Read the model definition and answer for the solid it produces. Units are mm, in the model's axes. Face numbers are marked on the shaded views. A direction names the side the tool comes from. Coordinates: 2 decimals unless noted, no trailing zeros. Order: outer loops, then holes, each group sorted by start corner. A loop starts at its lowest first (then second) coordinate and runs counter-clockwise, first axis right, second up.
from build123d import *

# Parameters (mm, degrees)
EXTRUDE_1_DEPTH     = 26
FILLET_1_R          = 1
FILLET_2_R          = 3
SKETCH_2_R          = 1.5
SKETCH_2_R_2        = 4
CUT_EXTRUDE_1_DEPTH = 26
SKETCH_3_R          = 1.5
SKETCH_3_R_2        = 4
CUT_EXTRUDE_2_DEPTH = 26


with BuildPart() as part:
    # 草图1 → 凸台-拉伸1 (new body)
    with BuildSketch(Plane.XY):
        Polygon((-19, -15), (19, -15), (19, 15), (17, 15), (17, -13), (-19, -13), align=None)
    extrude(amount=EXTRUDE_1_DEPTH)

    # 圆角1
    fillet_1_edges = [part.edges().sort_by_distance(p)[0] for p in [
        (17, -13, 13),
    ]]
    fillet(fillet_1_edges, radius=FILLET_1_R)

    # 圆角2
    fillet_2_edges = [part.edges().sort_by_distance(p)[0] for p in [
        (19, -15, 13),
    ]]
    fillet(fillet_2_edges, radius=FILLET_2_R)

    # 草图2 → 切除-拉伸1 (cut)
    with BuildSketch(Plane.ZY.offset(-17)):
        with BuildLine():
            Line((26, 15), (13, 15))
            ThreePointArc((13, 15), (22.192388155, 11.192388155), (26, 2))
            Line((26, 2), (26, 15))
        make_face()
        with BuildLine():
            Line((0, 15), (0, 2))
            ThreePointArc((0, 2), (3.807611845, 11.192388155), (13, 15))
            Line((13, 15), (0, 15))
        make_face()
        with Locations((6, 2)):
            Circle(SKETCH_2_R)
        with Locations((13, 9)):
            Circle(SKETCH_2_R)
        with Locations((13, -5)):
            Circle(SKETCH_2_R)
        with Locations((20, 2)):
            Circle(SKETCH_2_R)
        with Locations((13, 2)):
            Circle(SKETCH_2_R_2)
    extrude(amount=-CUT_EXTRUDE_1_DEPTH, mode=Mode.SUBTRACT)

    # 草图3 → 切除-拉伸2 (cut)
    with BuildSketch(Plane(origin=(0, -13, 0), x_dir=(1, 0, 0), z_dir=(0, 1, 0))):
        with BuildLine():
            ThreePointArc((-19, -13), (-15.192388155, -3.807611845), (-6, 0))
            Line((-6, 0), (-19, 0))
            Line((-19, 0), (-19, -13))
        make_face()
        with Locations(Location((-6, -6, 0), (0, 0, 270))):
            Circle(SKETCH_3_R)
        with Locations(Location((-6, -13, 0), (0, 0, 270))):
            Circle(SKETCH_3_R_2)
        with Locations(Location((1, -13, 0), (0, 0, 270))):
            Circle(SKETCH_3_R)
        with Locations(Location((-13, -13, 0), (0, 0, 270))):
            Circle(SKETCH_3_R)
        with Locations(Location((-6, -20, 0), (0, 0, 270))):
            Circle(SKETCH_3_R)
        with BuildLine():
            ThreePointArc((-6, -26), (-15.192388155, -22.192388155), (-19, -13))
            Line((-19, -13), (-19, -26))
            Line((-19, -26), (-6, -26))
        make_face()
    extrude(amount=-CUT_EXTRUDE_2_DEPTH, mode=Mode.SUBTRACT)


solid = part.part
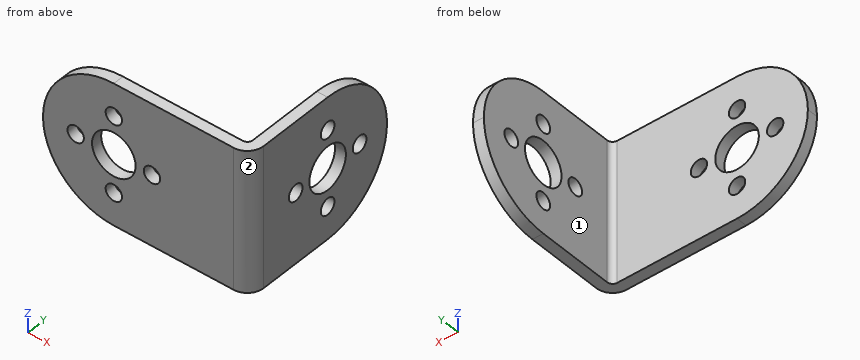
Q1. The part is cut by section C-C, the plane y = -5. Determine the outline of the cut face in (x, z).
Q2. The part is cut by section D-D, the plane z = 3.5. Determine the outline of the cut face in (x, y), then the cut area to 3 significant figures.
Q3. Each of these flat-tipped pins is pushed along its axis until it touches: P1, Ø5, axis at y = 2, z = 20, coming from the -X side; P2, Ø6, axis at x = -9.5, z = 18.5, coming from the +Y side. Where does it stop, or does it pass through?
Q4. Straight lines are drawn through the part: L1, parallel to Y at x = 17.55, z = 13; L2, parallel to X at y = 0.5, z = 20.75; L3, parallel to Y at x = 7.5, z = 24.25. For each, find the intervals that lie inside material, in ascending order.
Q5. The part is cut by section B-B, the plane z = 10.25. Determine the outline of the cut face in (x, y).
Q6. Which of the six approach directions +Z, -Z, +X, -X, +Y, -Y give full straight-line access (tool end or side, diameter ignored) to the marked faces 1 and 2?
Q7. The part is cut by section A-A, the plane x = 1. Determine the outline of the cut face in (y, z), then the cut area to 3 significant figures.
Computed values:
1. outline: (17, 0) - (19, 0) - (19, 11.5) - (17, 11.5) - close; (17, 14.5) - (19, 14.5) - (19, 26) - (17, 26) - close
2. outline: (-14.87, -15) - (16, -15) arc R3 ccw to (19, -12) - (19, 10.87) - (17, 10.87) - (17, -12) arc R1 cw to (16, -13) - (-14.87, -13) - close
2. area: 114 mm2
3. P1: stops at x = 17
3. P2: stops at y = -13
4. L1: y = -14.57 to -6.5, -3.5 to -2, 6 to 7.5, 10.5 to 15
4. L2: x = 17 to 19
4. L3: y = -15 to -13
5. outline: (-18.71, -15) - (-8.9, -15) - (-8.9, -13) - (-18.71, -13) - close; (-3.1, -15) - (16, -15) arc R3 ccw to (19, -12) - (19, -0.9) - (17, -0.9) - (17, -12) arc R1 cw to (16, -13) - (-3.1, -13) - close; (17, 4.9) - (19, 4.9) - (19, 14.71) - (17, 14.71) - close
6. face 1: +Z, -Z, -X, +Y
6. face 2: +Z, -Z, +X, -Y
7. outline: (-15, 0) - (-13, 0) - (-13, 11.5) - (-15, 11.5) - close; (-15, 14.5) - (-13, 14.5) - (-13, 26) - (-15, 26) - close
7. area: 46.0 mm2
